For this review, use the dimensioned drawing (mm, ordinates from the lowest corner) and the shaded views. Coordinates: 2 decimals unless noted, no trailing zeros. Order: outer loops, then holes, each group sorted by start corner. A loop starts at its lowest first (then second) coordinate and runs counter-clockwise, first axis right, second up. Notation, with made-up numbers: (-16.75, 55.25) -> (14.25, 55.25) arc R12 cw to (14.25, 59.25) -> close; hole circle Ø6 at (7, 5). An arc over 180 degrees is marked (long way). Return JSON: item names as keys, results as strings. Group by question number.
Item 1: For line 1 along Z through (x, y) = (31.75, 1.25); line 2 along X through (y, z) = (0.6, 9), list the stretches that pass through material, from the lowest coordinate up.
Item 2: Take a section at C-C (y = 1.65). Write out the cut boundary in (x, z), then the cut area to 3 significant figures.
Item 3: Take a section at A-A (z = 6.35). Write out the cut boundary in (x, y).
Item 4: Insertion check: pin 1 (5 mm diameter, centred on x = 31.75, z = 6.35, fed in from +Y). The pin has a flat end and moves straight along its axis. Give the tip position at first contact, or say it passes through.
Item 5: Take a section at B-B (x = 31.75). Write out the cut boundary in (y, z), then the cut area to 4 significant figures.
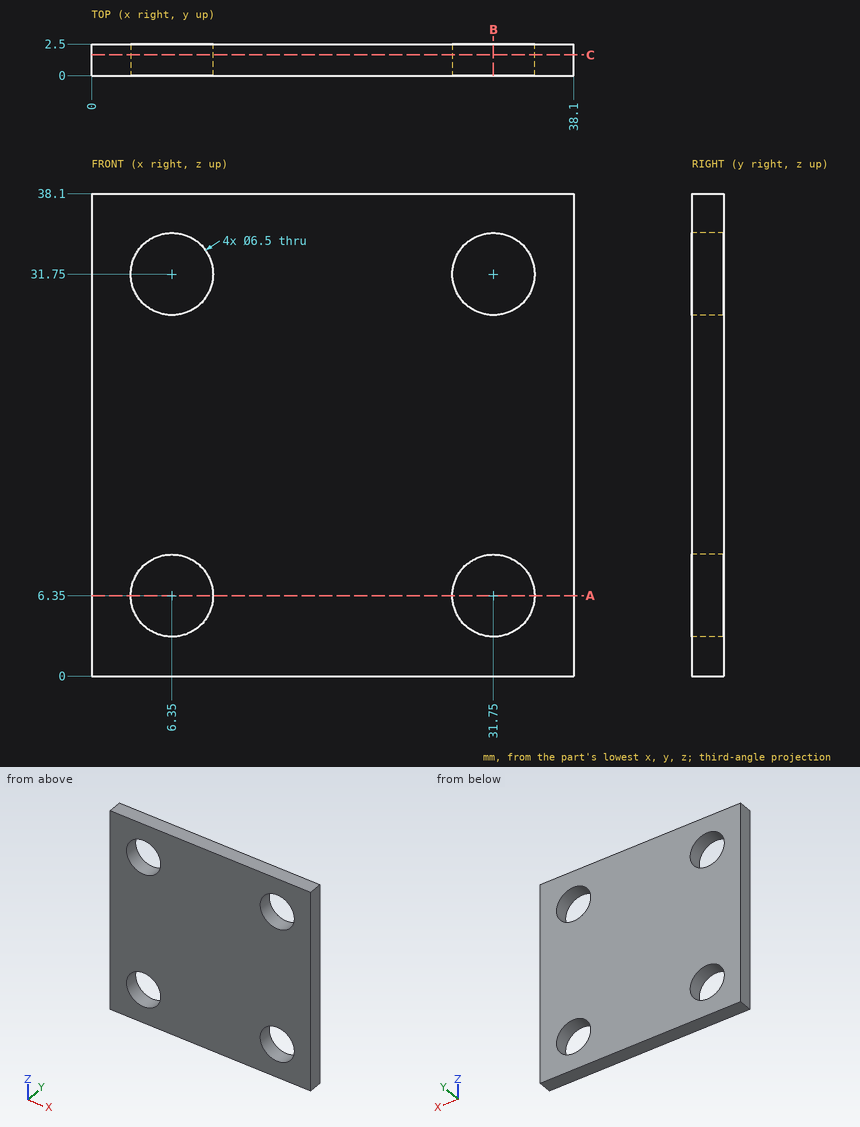
Findings below:
{
 "1": {"line 1": "z = 0 to 3.1, 9.6 to 28.5, 35 to 38.1", "line 2": "x = 0 to 4.47, 8.23 to 29.87, 33.63 to 38.1"},
 "2": {"outline": "(0, 0) -> (38.1, 0) -> (38.1, 38.1) -> (0, 38.1) -> close; hole circle Ø6.5 at (6.35, 6.35); hole circle Ø6.5 at (6.35, 31.75); hole circle Ø6.5 at (31.75, 6.35); hole circle Ø6.5 at (31.75, 31.75)", "area": "1,320 mm2"},
 "3": {"outline": "(0, 0) -> (3.1, 0) -> (3.1, 2.5) -> (0, 2.5) -> close; (9.6, 0) -> (28.5, 0) -> (28.5, 2.5) -> (9.6, 2.5) -> close; (35, 0) -> (38.1, 0) -> (38.1, 2.5) -> (35, 2.5) -> close"},
 "4": {"pin 1": "passes through"},
 "5": {"outline": "(0, 0) -> (2.5, 0) -> (2.5, 3.1) -> (0, 3.1) -> close; (0, 9.6) -> (2.5, 9.6) -> (2.5, 28.5) -> (0, 28.5) -> close; (0, 35) -> (2.5, 35) -> (2.5, 38.1) -> (0, 38.1) -> close", "area": "62.75 mm2"}
}
